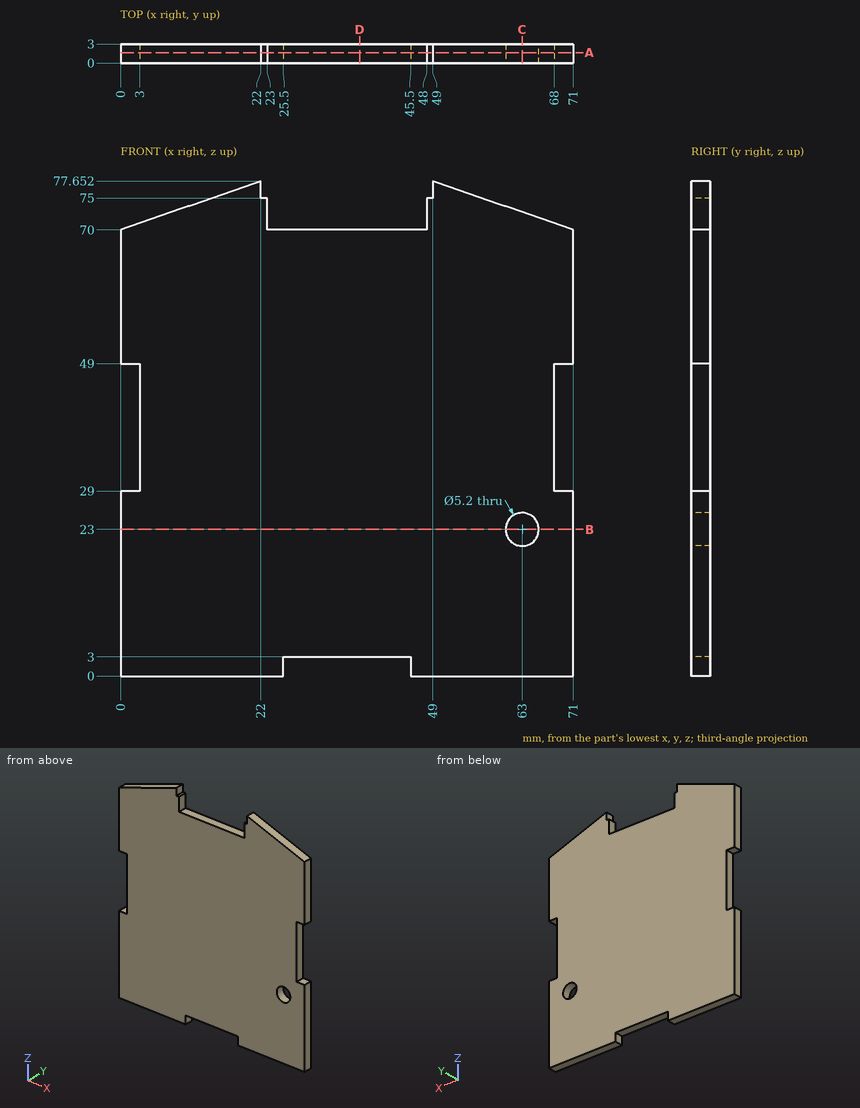
Verification items for this drawing (mm, ordinates from the low corner). Give positions to 0.01 mm unless a question says otherwise; leave off trailing zeros. Write each loop counter-clockwise with the first axis right and the second up, starting at its lowest first coordinate (ties: lowest second). Pieces come first, ordered by that corner, then holes. Notation, with made-up numbers: (-30.75, 35.25) -> (-12.75, 35.25) arc R22 cw to (-12.75, 44.25) -> close; hole circle Ø4 at (-31.5, 83). An arc over 180 degrees is marked (long way). Use CSV: the item, a comma, the result in double quotes.
(1) Sectioned sample at C-C (x = 63). Record the cut outline in (y, z).
Derived:
outline,"(0, 0) -> (3, 0) -> (3, 20.4) -> (0, 20.4) -> close; (0, 25.6) -> (3, 25.6) -> (3, 72.78) -> (0, 72.78) -> close"
(2) Sectioned sample at D-D (x = 37.5). Record the cut outline in (y, z), plus the area to 3 significant figures.
Derived:
outline,"(0, 3) -> (3, 3) -> (3, 70) -> (0, 70) -> close"
area,"201 mm^2"
(3) Sectioned sample at A-A (y = 1.65). Record the cut outline in (x, z), plus the area to 3 significant figures.
Derived:
outline,"(0, 0) -> (25.5, 0) -> (25.5, 3) -> (45.5, 3) -> (45.5, 0) -> (71, 0) -> (71, 29) -> (68, 29) -> (68, 49) -> (71, 49) -> (71, 70) -> (49, 77.65) -> (49, 75) -> (48, 75) -> (48, 70) -> (23, 70) -> (23, 75) -> (22, 75) -> (22, 77.65) -> (0, 70) -> (0, 49) -> (3, 49) -> (3, 29) -> (0, 29) -> close; hole circle Ø5.2 at (63, 23)"
area,"4,950 mm^2"
(4) Go/stop test with flat-tipped pins: pin 1 (0.5 mm diameter, centred on x = 22.5, y = 1.5, fed in from +Z); pin 2 (1.5 mm diameter, centred on y = 1.5, z = 1, fed in from -X); pin 3 (3 mm diameter, centred on x = 63, z = 23, fed in from +Y); pin 4 (1.5 mm diameter, centred on x = 1, y = 1, fed in from +Z). Record where each tip stops, or that it passes through.
Derived:
pin 1,"stops at z = 75"
pin 2,"stops at x = 0"
pin 3,"passes through"
pin 4,"stops at z = 70.61"
(5) Material ranges on L1, parallel to X at y = 1.7, z = 33; L2, parallel to Z at x = 32, y = 0.5; L3, parallel to Z at x = 63, y = 1.05, recorded low to high.
Derived:
L1,"x = 3 to 68"
L2,"z = 3 to 70"
L3,"z = 0 to 20.4, 25.6 to 72.78"
(6) Sectioned sample at B-B (z = 23). Record the cut outline in (x, y), plus the area to 3 significant figures.
Derived:
outline,"(0, 0) -> (60.4, 0) -> (60.4, 3) -> (0, 3) -> close; (65.6, 0) -> (71, 0) -> (71, 3) -> (65.6, 3) -> close"
area,"197 mm^2"
